For this review, use the dimensioned drawing (mm, ordinates from the lowest corner) and the shaded views. A direction names the side the tool comes from. Round coordinates to 2 decimals unless told otherwise and drop trailing zeros. Order: outer loops, then holes, each group sorted by start corner. A loop starts at its lowest first (then second) coordinate and runs counter-clockwise, first axis right, second up. Notation, with made-up numbers: (24, 67.25) -> (81, 67.25) arc R20 cw to (81, 78.25) -> close; hole circle Ø10 at (4.5, 78.25). An arc over 180 degrees is marked (long way). Answer in a Markdown table with one row per item.
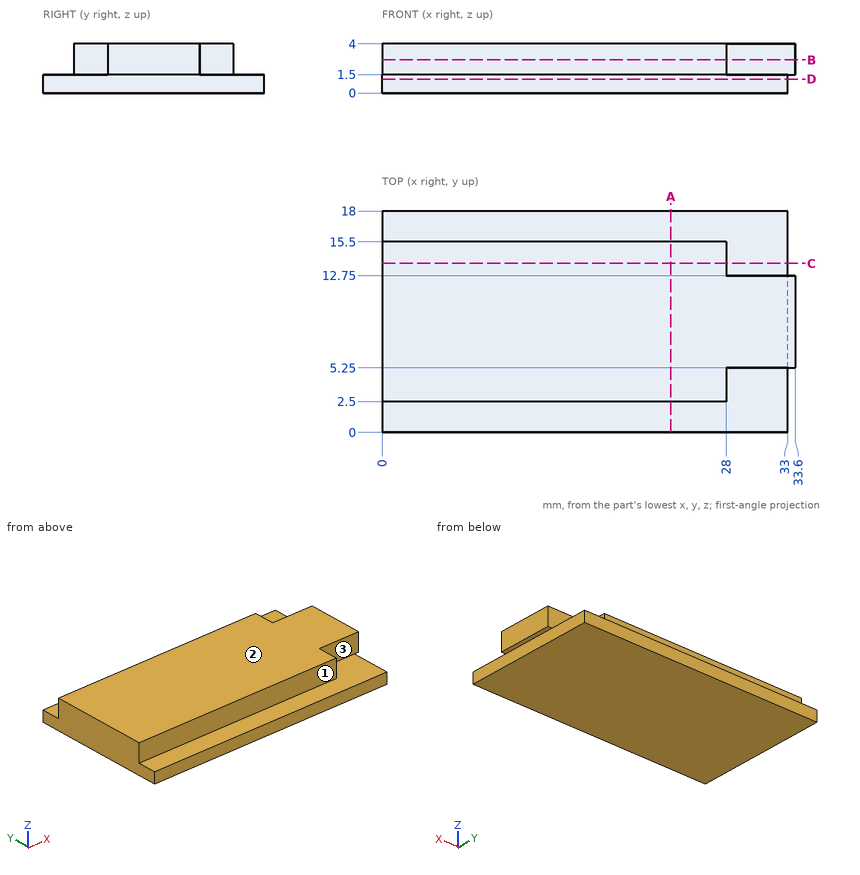
Q1. To check wall thickness, follow probe 1 along X at (y, z) = (10.25, 1.15); probe 2 along Z at (x, y) = (18, 1); probe 3 along Y at (x, z) = (11, 1.65). State the ranges of each line that lie inside material, in increasing order.
Answer key:
| item | result |
|---|---|
| probe 1 | x = 0 to 33 |
| probe 2 | z = 0 to 1.5 |
| probe 3 | y = 2.5 to 15.5 |
Q2. Take a section at D-D, the plane z = 1.15. Write out the cut boundary in (x, y).
Answer key:
| item | result |
|---|---|
| outline | (0, 0) -> (33, 0) -> (33, 18) -> (0, 18) -> close |
Q3. Take a section at B-B, the plane z = 2.7. Write out the cut boundary in (x, y), then the cut area to 3 significant figures.
Answer key:
| item | result |
|---|---|
| outline | (0, 2.5) -> (28, 2.5) -> (28, 5.25) -> (33.6, 5.25) -> (33.6, 12.75) -> (28, 12.75) -> (28, 15.5) -> (0, 15.5) -> close |
| area | 406 mm^2 |
Q4. Take a section at A-A, the plane x = 23.5. Write out the cut boundary in (y, z), then the cut area to 3 significant figures.
Answer key:
| item | result |
|---|---|
| outline | (0, 0) -> (18, 0) -> (18, 1.5) -> (15.5, 1.5) -> (15.5, 4) -> (2.5, 4) -> (2.5, 1.5) -> (0, 1.5) -> close |
| area | 59.5 mm^2 |
Q5. Tool access review of the marked faces 1, 2 and 3: name each direction out of +Z, -Z, +X, -X, +Y, -Y from which nothing blocks a thin tool from reaching the whole face with its end or side.
Answer key:
| item | result |
|---|---|
| face 1 | +Z, +X, -X, -Y |
| face 2 | +Z, +X, -X, +Y, -Y |
| face 3 | +Z, +X, -Y |
Q6. Take a section at C-C, the plane y = 13.75. Write out the cut boundary in (x, z).
Answer key:
| item | result |
|---|---|
| outline | (0, 0) -> (33, 0) -> (33, 1.5) -> (28, 1.5) -> (28, 4) -> (0, 4) -> close |
Q7. Clearance check with flat-ended pins moving along their axes: pin 1 Ø1 at (x, z) = (4.5, 2.5) entering from -Y; pin 2 Ø0.8 at (y, z) = (14, 3) entering from +X; pin 3 Ø0.8 at (y, z) = (6.5, 0.5) entering from +X. State where each tip first meets the part, or that it passes through.
Answer key:
| item | result |
|---|---|
| pin 1 | stops at y = 2.5 |
| pin 2 | stops at x = 28 |
| pin 3 | stops at x = 33 |
